Geometry check sheet. Reference: the model listing, model coordinates, mm. Face numbers are marked on the shaded views. A direction names the side the tool comes from. Round coordinates to 2 decimals unless told otherwise and drop trailing zeros. Write each loop counter-clockwise with the first axis right and the second up, starting at its lowest first coordinate (ties: lowest second). Pieces come first, ordered by that corner, then holes. Notation, with made-up numbers: (-9, 54) - (31, 54) arc R22 ccw to (31, 67) - close; hole circle Ø8 at (-31.5, 80). An arc over 180 degrees is marked (long way). Return JSON: item names as keys, results as strings.
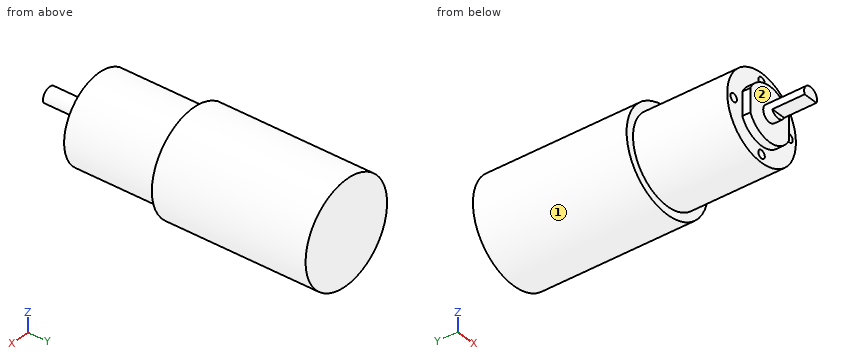
```python
from build123d import *

# Parameters (mm, degrees)
BOSS_EXTRUDE1_DEPTH = 12
BOSS_EXTRUDE2_DEPTH = 3.2
BOSS_EXTRUDE3_DEPTH = 3
SKETCH6_R           = 16
BOSS_EXTRUDE4_DEPTH = 35
SKETCH7_R           = 19
BOSS_EXTRUDE5_DEPTH = 57.1
SKETCH8_R           = 1.5
CUT_EXTRUDE1_DEPTH  = 10


with BuildPart() as part:
    # Sketch2 → Boss-Extrude1 (new body)
    with BuildSketch(Plane(origin=(0, 0, 0), x_dir=(1, 0, 0), z_dir=(0, 1, 0))):
        with BuildLine():
            Line((2.75, 1.198957881), (-2.75, 1.198957881))
            ThreePointArc((-2.75, 1.198957881), (-0.612372436, -2.936835031), (3, 0))
            ThreePointArc((3, 0), (2.936835031, 0.612372436), (2.75, 1.198957881))
        make_face()
    extrude(amount=BOSS_EXTRUDE1_DEPTH)

    # Sketch3 → Boss-Extrude2 (add)
    with BuildSketch(Plane(origin=(0, 12, 0), x_dir=(1, 0, 0), z_dir=(0, 1, 0))):
        with BuildLine():
            Line((2.75, 1.198957881), (-2.75, 1.198957881))
            ThreePointArc((-2.75, 1.198957881), (-0.612372436, -2.936835031), (3, 0))
            ThreePointArc((3, 0), (2.936835031, 0.612372436), (2.75, 1.198957881))
        make_face()
        with BuildLine():
            ThreePointArc((2.75, 1.198957881), (0, 3), (-2.75, 1.198957881))
            Line((-2.75, 1.198957881), (2.75, 1.198957881))
        make_face()
        with BuildLine():
            ThreePointArc((-2.75, 1.198957881), (0, -3), (2.75, 1.198957881))
            Line((2.75, 1.198957881), (-2.75, 1.198957881))
        make_face()
    extrude(amount=BOSS_EXTRUDE2_DEPTH)

    # Sketch5 → Boss-Extrude3 (add)
    with BuildSketch(Plane(origin=(0, 15.2, 0), x_dir=(1, 0, 0), z_dir=(0, 1, 0))):
        with BuildLine():
            Line((-9, 4.358898944), (-9, -4.358898944))
            ThreePointArc((-9, -4.358898944), (0, -10), (9, -4.358898944))
            Line((9, -4.358898944), (9, 4.358898944))
            ThreePointArc((9, 4.358898944), (0, 10), (-9, 4.358898944))
        make_face()
    extrude(amount=BOSS_EXTRUDE3_DEPTH)

    # Sketch6 → Boss-Extrude4 (add)
    with BuildSketch(Plane(origin=(0, 18.2, 0), x_dir=(1, 0, 0), z_dir=(0, 1, 0))):
        Circle(SKETCH6_R)
    extrude(amount=BOSS_EXTRUDE4_DEPTH)

    # Sketch7 → Boss-Extrude5 (add)
    with BuildSketch(Plane(origin=(0, 53.2, 0), x_dir=(1, 0, 0), z_dir=(0, 1, 0))):
        Circle(SKETCH7_R)
    extrude(amount=BOSS_EXTRUDE5_DEPTH)

    # Sketch8 → Cut-Extrude1 (cut)
    with BuildSketch(Plane.XZ.offset(-18.2)):
        with Locations((0, 13)):
            Circle(SKETCH8_R)
        with Locations((13, 0)):
            Circle(SKETCH8_R)
        with Locations((0, -13)):
            Circle(SKETCH8_R)
        with Locations((-13, 0)):
            Circle(SKETCH8_R)
    extrude(amount=-CUT_EXTRUDE1_DEPTH, mode=Mode.SUBTRACT)


solid = part.part
```
(1) Section check A-A, the plane z = 0. Enter the section's corners in (x, y), plus the area to 4 significant figures.
Response values:
{"outline": "(-19, 53.2) - (-16, 53.2) - (-16, 18.2) - (-14.5, 18.2) - (-14.5, 28.2) - (-11.5, 28.2) - (-11.5, 18.2) - (-9, 18.2) - (-9, 15.2) - (-3, 15.2) - (-3, 0) - (3, 0) - (3, 15.2) - (9, 15.2) - (9, 18.2) - (11.5, 18.2) - (11.5, 28.2) - (14.5, 28.2) - (14.5, 18.2) - (16, 18.2) - (16, 53.2) - (19, 53.2) - (19, 110.3) - (-19, 110.3) - close", "area": "3,375 mm^2"}
(2) Access from +Z, -Z, +X, -X, +Y, -Y to the whole of each face (thin tool, end or side, straight path). Record for the marked faces 1 and 2.
Response values:
{"face 1": "+Y, -Y", "face 2": "-Y"}
(3) Material ranges on line 1 along Z through (x, y) = (0, 21.5); line 2 along Y through (x, z) = (2.5, 4.5); line 3 along Y through (x, z) = (2.5, 10.5), recorded low to high. Write a range as [from, to].
Response values:
{"line 1": "z = [-16, -14.5], [-11.5, 11.5], [14.5, 16]", "line 2": "y = [15.2, 110.3]", "line 3": "y = [18.2, 110.3]"}
(4) Section check C-C, the plane y = 93. Enter the section's corners in (x, z), plus the area to 3 significant figures.
Response values:
{"outline": "circle Ø38 at (0, 0)", "area": "1,130 mm^2"}
(5) Section check D-D, the plane z = 13. Enter the section's corners in (x, y), plus the area to 3 significant figures.
Response values:
{"outline": "(-13.86, 53.2) - (-9.33, 53.2) - (-9.33, 18.2) - (-1.5, 18.2) - (-1.5, 28.2) - (1.5, 28.2) - (1.5, 18.2) - (9.33, 18.2) - (9.33, 53.2) - (13.86, 53.2) - (13.86, 110.3) - (-13.86, 110.3) - close", "area": "2,210 mm^2"}
(6) Gauge pin test, flat ends, axial feed: pin 1 (3 mm diameter, centred on x = -4, z = -5, fed in from -Y); pin 2 (3.5 mm diameter, centred on x = 0, z = 13, fed in from -Y); pin 3 (2 mm diameter, centred on x = 5, y = 85, fed in from +Z). Record the tip position at first contact, or that the pin passes through.
Response values:
{"pin 1": "stops at y = 15.2", "pin 2": "stops at y = 18.2", "pin 3": "stops at z = 18.57"}
(7) Section check B-B, the plane x = 0. Enter the section's corners in (y, z), plus the area to 3 significant figures.
Response values:
{"outline": "(0, -1.2) - (12, -1.2) - (12, -3) - (15.2, -3) - (15.2, -10) - (18.2, -10) - (18.2, -11.5) - (28.2, -11.5) - (28.2, -14.5) - (18.2, -14.5) - (18.2, -16) - (53.2, -16) - (53.2, -19) - (110.3, -19) - (110.3, 19) - (53.2, 19) - (53.2, 16) - (18.2, 16) - (18.2, 14.5) - (28.2, 14.5) - (28.2, 11.5) - (18.2, 11.5) - (18.2, 10) - (15.2, 10) - (15.2, 3) - (0, 3) - close", "area": "3,360 mm^2"}
